Build history of the part. All positions in model axes, mm. Face numbers are marked on the shaded views. A direction names the side the tool comes from. Round coordinates to 2 decimals unless told otherwise and drop trailing zeros. Order: outer loops, then holes, each group sorted by start corner. A loop starts at its lowest first (then second) coordinate and runs counter-clockwise, first axis right, second up. Notation, with made-up numbers: (28.5, 1) -> (59.5, 1) arc R27 cw to (59.5, 35) -> close; hole circle Ø2 at (76, -5.75). An arc over 180 degrees is marked (long way). Write item = value, one per line.
from build123d import *

# Parameters (mm, degrees)
EXTRUDE_1_DEPTH = 100
EXTRUDE_2_DEPTH = 240
SKETCH_1_4_W    = 30
SKETCH_1_4_H    = 35
SKETCH_1_4_R    = 5
EXTRUDE_3_DEPTH = 30


with BuildPart() as part:
    # Эскиз1 → Бобышка-Вытянуть1 (new body)
    with BuildSketch(Plane.XY):
        Polygon((0, 60), (0, 0), (860, 0), (860, 60), (860, 95), (860, 630), (820, 630), (820, 40), (40, 40), (40, 630), (0, 630), (0, 95), align=None)
    extrude(amount=EXTRUDE_1_DEPTH)

    # Эскиз1<3> → Бобышка-Вытянуть2 (add)
    with BuildSketch(Plane.XY):
        Polygon((0, 765), (0, 630), (40, 630), (820, 630), (860, 630), (860, 765), (860, 800), (0, 800), align=None)
    extrude(amount=EXTRUDE_2_DEPTH)

    # Эскиз1<4> → Бобышка-Вытянуть3 (add)
    # profile 1 of 4: a face of its own
    with BuildSketch(Plane.XY):
        with Locations((-15, 77.5)):
            Rectangle(SKETCH_1_4_W, SKETCH_1_4_H)
        with Locations((-20, 77.5)):
            Circle(SKETCH_1_4_R, mode=Mode.SUBTRACT)
    # profile 2 of 4: a face of its own
    with BuildSketch(Plane.XY):
        with Locations((875, 77.5)):
            Rectangle(SKETCH_1_4_W, SKETCH_1_4_H)
        with Locations((880, 77.5)):
            Circle(SKETCH_1_4_R, mode=Mode.SUBTRACT)
    # profile 3 of 4: a face of its own
    with BuildSketch(Plane.XY):
        with Locations((-15, 782.5)):
            Rectangle(SKETCH_1_4_W, SKETCH_1_4_H)
        with Locations((-20, 782.720518287)):
            Circle(SKETCH_1_4_R, mode=Mode.SUBTRACT)
    # profile 4 of 4: a face of its own
    with BuildSketch(Plane.XY):
        with Locations((875, 782.5)):
            Rectangle(SKETCH_1_4_W, SKETCH_1_4_H)
        with Locations((880, 782.5)):
            Circle(SKETCH_1_4_R, mode=Mode.SUBTRACT)
    extrude(amount=EXTRUDE_3_DEPTH)


solid = part.part
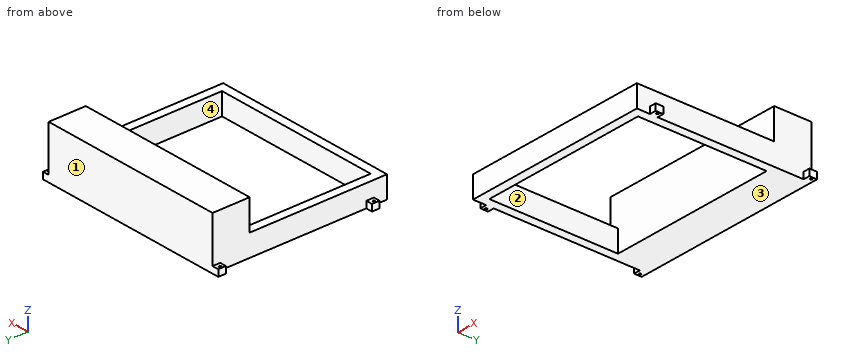
Q1. Cut at C-C, the plane y = 543.5. List the corners of the cut face in (x, z).
Check values:
outline = (0, 0) -> (40, 0) -> (40, 100) -> (0, 100) -> close; (820, 0) -> (860, 0) -> (860, 100) -> (820, 100) -> close
Q2. Mould opens along X. For the marked faces 3 and 4 say: released by +X, released by -X, zero draft, split by the parting line, or undercut.
Check values:
face_3 = zero draft
face_4 = undercut
Q3. Cut at B-B, the plane x = 722. List the corners of the cut face in (y, z).
Check values:
outline = (0, 0) -> (40, 0) -> (40, 100) -> (0, 100) -> close; (630, 0) -> (800, 0) -> (800, 240) -> (630, 240) -> close
Q4. Which spindle directions (+Z, -Z, +X, -X, +Y, -Y) get a long thin tool onto all of the face, cutting with end or side? Do the marked faces 1 and 2. Say none if no direction does.
Check values:
face_1 = +Z, -Z, +X, -X, +Y
face_2 = +Z, -Z
Q5. Cut at D-D, the plane y = 674.5. List the corners of the cut face in (x, z).
Check values:
outline = (0, 0) -> (860, 0) -> (860, 240) -> (0, 240) -> close
Q6. Probe probe 1 along X at (y, z) = (77, 11); probe 2 along Y at (x, z) = (880, 12.5); probe 3 along Y at (x, z) = (-20, 8). List the from-to ranges inside material, lowest first.
Check values:
probe_1 = -30 to -24.97, -15.03 to 40, 820 to 875.03, 884.97 to 890
probe_2 = 60 to 72.5, 82.5 to 95, 765 to 777.5, 787.5 to 800
probe_3 = 60 to 72.5, 82.5 to 95, 765 to 777.72, 787.72 to 800
Q7. Flat gauge pins, fed straight in: pin 1 (24 mm diameter, centred on x = 875.5, y = 84.5, fed in from +Z); pin 2 (6 mm diameter, centred on x = 117, z = 114.5, fed in from -Y); pin 3 (24 mm diameter, centred on x = -15.5, z = 10.5, fed in from -Y); pin 4 (9 mm diameter, centred on x = 880, y = 782.5, fed in from +Z). Where does each tip first touch, or does it go through?
Check values:
pin_1 = 30
pin_2 = 630
pin_3 = 60
pin_4 = through
Q8. Cut at A-A, the plane z = 90. List the corners of the cut face in (x, y).
Check values:
outline = (0, 0) -> (860, 0) -> (860, 800) -> (0, 800) -> close; hole (40, 40) -> (820, 40) -> (820, 630) -> (40, 630) -> close
